Can you work these out from the model? Positions are in its coordinate system, mm. Face numbers are marked on the shaded views. A direction names the side the tool comes from. Give positions to 0.01 mm unless a question says otherwise; leave off trailing zeros. Loops run counter-clockwise (first coordinate to the right, second up) from the corner with the lowest first, then second, coordinate; pieces in that order, holes last. Notation, with made-up numbers: (22.5, -11) - (44.5, -11) arc R14 cw to (44.5, 13) - close; hole circle Ø5 at (42.5, 7.5). An arc over 180 degrees is marked (long way). Answer as a JSON object with one key per item and string values. Group by question number.
Item 1: Suppose I cut it at C-C on z = 147.6. Write out the boundary of the cut face in (x, y), and give its area (3 significant figures).
Item 2: Suppose I cut it at B-B on x = -35. Write out the boundary of the cut face in (y, z), and give its area (3 significant figures).
Item 3: Which directions (+Z, -Z, +X, -X, +Y, -Y) give clear straight access to the entire face, cutting with the end or side of a thin tool? Please do the marked faces 5, 6, 7, 8 and 9.
Item 4: Suppose I cut it at D-D on x = -28. Write out the boundary of the cut face in (y, z).
Item 5: Please list where these lines run through material, in increasing order: L1, parallel to Z at x = -28, y = 12.5; L2, parallel to Z at x = -42, y = 10; L3, parallel to X at y = 10, z = 139.
Item 6: Will these pins go through, and if not, where does the flat tip stop? pin 1 (3 mm diameter, centred on x = -50.5, z = 117.5, fed in from -Y); pin 2 (4 mm diameter, centred on x = -29, y = -11.5, fed in from +Z); pin 3 (1.8 mm diameter, centred on x = -33.5, z = 96, fed in from +Y); pin 4 (2.5 mm diameter, centred on x = -28, z = 163.6, fed in from -Y).
Item 7: Thinking about a two-plate mould opening in X: for the marked faces 1, 2, 3 and 4, which applies, pulls with the +X half, pulls with the -X half, needs draft (parallel to the pull), parting line crosses it, or undercut?
Item 8: Suppose I cut it at A-A on y = -7. Write out the boundary of the cut face in (x, z).
Autodesk Inventor part; units mm, degrees
ref_plane "YZ Plane" through (0, 0, 0) normal (1, 0, 0) x (0, 1, 0)
ref_plane "XZ Plane" through (0, 0, 0) normal (0, 1, 0) x (-1, 0, 0)
ref_plane "XY Plane" through (0, 0, 0) normal (0, 0, 1) x (1, 0, 0)
sketch "Sketch1" plane through (0, 0, 0) normal (0, 1, 0) x (-1, 0, 0)
  line L0 (0, 0) -> (0, 62)
  line L1 (0, 62) -> (70, 62)
  line L2 (70, 62) -> (70, 0)
  line L3 (76, 0) -> (76, 68)
  line L4 (76, 68) -> (-6, 68)
  line L5 (-6, 68) -> (-6, 0)
  line L6 (70, 0) -> (76, 0)
  line L7 (-6, 0) -> (0, 0)
  dimension "d0" = 62
  dimension "d1" = 70
  dimension "d2" = 6
  dimension "d5" = 62
extrude "Extrusion1" add sketch "Sketch1" along normal blind 40
sketch "Sketch2" plane through (6, 0, 68) normal (1, 0, 0) x (0, 0, -1)
  line L0 (68, 0) -> (68, 40)
  circle A0 centre (56, 25) radius 1.5
  circle A1 centre (51, 20) radius 1.5
  circle A2 centre (56, 15) radius 1.5
  circle A3 centre (61, 20) radius 1.5
  point P0 (56, 20)
  dimension "d9" = 3
  dimension "d12" = 360
extrude "Extrusion2" cut sketch "Sketch2" against normal up to surface (6 mm away)
sketch "Sketch3" plane through (-70, 0, 62) normal (1, 0, 0) x (0, 0, -1)
  line L0 (62, 0) -> (62, 40)
  line L1 (62, 20) -> (58, 20)
  circle A0 centre (50, 20) radius 5.75
  dimension "d16" = 4
  dimension "d18" = 11.5
extrude "Extrusion3" add sketch "Sketch3" along normal blind 5
fillet "Fillet1" radius 8 4 edges at (3, 40, 0) (3, 0, 0) (-73, 0, 0) (-73, 40, 0)
sketch "Sketch4" plane through (-76, 0, 68) normal (0, 0, 1) x (1, 0, 0)
  line L0 (41, 0) -> (41, 20)
  line L1 (30, 0) -> (30, 40)
  line L2 (76, 40) -> (6, 40)
  line L3 (52, 0) -> (52, 40)
  line L4 (25, 0) -> (25, 40)
  line L5 (57, 0) -> (57, 40)
  line L6 (25, 40) -> (30, 40)
  line L7 (52, 40) -> (57, 40)
  line L8 (52, 0) -> (57, 0)
  line L9 (76, 0) -> (6, 0)
  line L10 (30, 0) -> (25, 0)
  dimension "d22" = 11
  dimension "d23" = 11
  dimension "d24" = 5
  dimension "d25" = 5
extrude "Extrusion4" add sketch "Sketch4" along normal blind 24 contours L9 L4 L2 L1 | L2 L5 L8 L3
sketch "Sketch5" plane through (-76, 0, 92) normal (0, 0, 1) x (1, 0, 0)
  line L0 (25, 0) -> (25, 40)
  line L1 (57, 0) -> (57, 40)
  line L2 (25, 0) -> (57, 0)
  line L3 (57, 0) -> (57, 40)
  line L4 (52, 0) -> (52, 40)
  line L5 (57, 40) -> (52, 40)
  line L6 (30, 0) -> (52, 0)
  line L7 (41, 3.3) -> (41, 9.3)
  line L8 (41, 9.3) -> (52, 9.3)
  line L9 (41, 9.3) -> (30, 9.3)
  line L10 (52, 9.3) -> (52, 40)
  line L11 (76, 40) -> (6, 40)
  line L12 (30, 40) -> (30, 0)
  line L13 (30, 9.3) -> (30, 40)
  line L14 (30, 40) -> (25, 40)
  line L15 (25, 40) -> (25, 0)
  line L16 (76, 0) -> (6, 0)
  dimension "d29" = 6
extrude "Extrusion5" add sketch "Sketch5" along normal blind 6 contours L0 L11 L12 L2 | L12 L9 L8 L4 L2 | L4 L5 L1 L2
sketch "Sketch6" plane through (-76, 0, 98) normal (0, 0, 1) x (1, 0, 0)
  line L0 (25, 0) -> (25, 40)
  line L1 (25, 40) -> (25, 0)
  line L2 (57, 40) -> (57, 0)
  line L3 (25, 0) -> (57, 0)
  line L4 (57, 0) -> (57, 40)
  line L5 (52, 0) -> (52, 40)
  line L6 (57, 40) -> (52, 40)
  line L7 (30, 40) -> (25, 40)
  line L8 (25, 40) -> (30, 40)
  line L9 (30, 0) -> (52, 0)
  line L10 (30, 40) -> (30, 0)
  line L11 (30, 0) -> (52, 0)
  line L12 (52, 40) -> (52, 9.3)
  line L13 (52, 40) -> (52, 0)
  line L14 (25, 0) -> (57, 0)
  point P0 (76, 0)
extrude "Extrusion6" add sketch "Sketch6" along normal blind 13.8
sketch "Sketch8" plane through (-76, 0, 111.8) normal (0, 0, 1) x (1, 0, 0)
  line L0 (52, 9.3) -> (30, 9.3)
  arc A0 (30.0455, 19.3) -> (51.9545, 19.3) centre (41, 20.3) ccw
  line L1 (51.9545, 19.3) -> (52, 19.3)
  line L2 (52, 0) -> (52, 40)
  line L3 (30, 40) -> (52, 40)
  line L4 (52, 19.3) -> (52, 40)
  line L5 (57, 40) -> (52, 40)
  line L6 (52, 40) -> (57, 40)
  line L7 (57, 40) -> (57, 6.3)
  line L8 (57, 40) -> (57, 0)
  line L9 (57, 6.3) -> (25, 6.3)
  line L10 (25, 0) -> (25, 40)
  line L11 (0, 40) -> (25, 40)
  line L12 (25, 6.3) -> (25, 40)
  line L13 (25, 40) -> (30, 40)
  line L14 (30, 40) -> (30, 19.3)
  line L15 (30, 40) -> (30, 0)
  line L16 (30, 19.3) -> (30.0455, 19.3)
  point P0 (76, 0)
  dimension "d37" = 33.7
  dimension "d38" = 11
extrude "Extrusion7" add sketch "Sketch8" along normal blind 13.8 contours L2 L9 L15 L0 | L0 A0 L1 L2 | L2 L5 L7 L9 | L0 L15 L16 A0 | L15 L9 L10 L13 L14
sketch "Sketch9" plane through (-76, 0, 125.6) normal (0, 0, 1) x (1, 0, 0)
  line L0 (25, 6.3) -> (57, 6.3)
  arc A0 (30.0455, 19.3) -> (51.9545, 19.3) centre (41, 20.3) ccw
  arc A1 (38, 20.3) -> (44, 20.3) centre (41, 20.3) ccw
  line L1 (25, 40) -> (25, 6.3)
  line L2 (25, 6.3) -> (25, 40)
  line L3 (57, 6.3) -> (57, 40)
  line L4 (25, 40) -> (57, 40)
  line L5 (38, 20.3) -> (30, 20.3)
  line L6 (30, 19.3) -> (30, 40)
  line L7 (44, 20.3) -> (52, 20.3)
  line L8 (52, 40) -> (52, 20.3)
  line L9 (52, 40) -> (57, 40)
  line L10 (57, 40) -> (57, 6.3)
  line L11 (57, 6.3) -> (25, 6.3)
  point P0 (76, 0)
  dimension "d41" = 6
extrude "Extrusion8" add sketch "Sketch9" along normal blind 50 contours L1 L4 L6 L5 A1 L7 L8 L3 L0
sketch "Sketch10" plane through (0, 40, 0) normal (0, 1, 0) x (1, 0, 0)
  line L0 (-24, -98) -> (-46, -98)
  line L1 (-46, -98) -> (-24, -98)
  line L2 (-24, -175.6) -> (-46, -175.6)
  line L3 (-19, -68) -> (-19, -175.6)
  line L4 (-19, -175.6) -> (-24, -175.6)
  line L5 (-24, -175.6) -> (-24, -98)
  line L6 (-24, -98) -> (-19, -98)
  line L7 (-19, -98) -> (-19, -175.6)
  line L8 (-51, -175.6) -> (-19, -175.6)
  line L9 (-51, -175.6) -> (-46, -175.6)
  line L10 (-46, -98) -> (-51, -98)
  line L11 (-51, -98) -> (-51, -175.6)
  point P0 (0, 0)
extrude "Extrusion9" cut sketch "Sketch10" against normal up to surface (19.7 mm away)
sketch "Sketch11" plane through (-76, 0, 175.6) normal (0, 0, 1) x (1, 0, 0)
  arc A0 (38, 20.3) -> (44, 20.3) centre (41, 20.3) ccw
  line L0 (52, 20.3) -> (44, 20.3)
  arc A1 (19.7397, 20.3) -> (62.2603, 20.3) centre (41, 20.3) ccw
  arc A2 (38, 20.3) -> (44, 20.3) centre (41, 20.3) ccw
  line L1 (19.7397, 20.3) -> (38, 20.3)
  line L2 (44, 20.3) -> (62.2603, 20.3)
  point P0 (76, 0)
extrude "Extrusion10" add sketch "Sketch11" along normal blind 36
sketch "Sketch12" plane through (-76, 0, 211.6) normal (0, 0, 1) x (1, 0, 0)
  arc A0 (38, 20.3) -> (44, 20.3) centre (41, 20.3) ccw
  circle A1 centre (41, 20.3) radius 19
  point P0 (76, 0)
  dimension "d49" = 38
extrude "Extrusion11" cut sketch "Sketch12" against normal blind 32
sketch "Sketch13" plane through (-76, 0, 211.6) normal (0, 0, 1) x (1, 0, 0)
  line L0 (62.2603, 20.3) -> (57, 20.3)
  arc A0 (19.7397, 20.3) -> (62.2603, 20.3) centre (41, 20.3) ccw
  line L1 (22, 20.3) -> (38, 20.3)
  arc A1 (22, 20.3) -> (60, 20.3) centre (41, 20.3) ccw
  arc A2 (22, 20.3) -> (60, 20.3) centre (41, 20.3) ccw
  line L2 (19.7397, 20.3) -> (22, 20.3)
  line L3 (62.2603, 20.3) -> (60, 20.3)
  point P0 (76, 0)
extrude "Extrusion12" add sketch "Sketch13" along normal blind 6.2
fillet "Fillet3" radius 1 5 edges at (-76, 20, 68) (-35, 40, 68) (-6.5, 40, 68) (-63.5, 40, 68) (6, 20, 68)
sketch "Sketch20" plane through (-19, 0, 111.8) normal (1, 0, 0) x (0, 0, -1)
  line L0 (0, 6.3) -> (-63.8, 6.3)
  line L1 (0, 6.3) -> (0, 0)
  line L2 (-63.8, 6.3) -> (0, 6.3)
  line L3 (0, 6.3) -> (0, 0)
  line L4 (0, 0) -> (-63.8, 0)
  line L5 (-63.8, 0) -> (-63.8, 6.3)
  point P0 (111.8, 0)
extrude "Extrusion19" add sketch "Sketch20" against normal up to surface (5 mm away)
sketch "Sketch21" plane through (-51, 0, 68) normal (-1, 0, 0) x (0, 0, 1)
  line L0 (43.8, 6.3) -> (107.6, 6.3)
  line L1 (0, 0) -> (107.6, 0)
  line L2 (43.8, 6.3) -> (107.6, 6.3)
  line L3 (107.6, 6.3) -> (107.6, 0)
  line L4 (107.6, 0) -> (43.8, 0)
  line L5 (43.8, 0) -> (43.8, 6.3)
  point P0 (-68, 0)
  point P1 (107.6, 6.3)
  point P2 (43.8, 0)
extrude "Extrusion20" add sketch "Sketch21" against normal up to surface (5 mm away)
sketch "Sketch22" plane through (-51, 20.3, 98) normal (-1, 0, 0) x (0, 0, 1)
  line L0 (-31, 19.7) -> (0, 19.7)
  line L1 (-31, 19.7) -> (0, 19.7)
  line L2 (0, 0) -> (27.6, 0)
  line L3 (0, 19.7) -> (0, 0)
  line L4 (77.6, 0) -> (119.8, 0)
  line L5 (0, 0) -> (77.6, 0)
  line L6 (-30, -20.3) -> (77.6, -20.3)
  line L7 (77.6, 0) -> (77.6, -20.3)
  line L8 (-31, 19.7) -> (-31, -20.3)
  line L9 (77.6, -20.3) -> (-31, -20.3)
  line L10 (-31, -20.3) -> (-31, 19.7)
  point P0 (-98, -20.3)
extrude "Extrusion21" add sketch "Sketch22" along normal up to surface (5.2603 mm away)
sketch "Sketch23" plane through (-19, 20.3, 98) normal (1, 0, 0) x (0, 0, -1)
  line L0 (31, 19.7) -> (0, 19.7)
  line L1 (0, 19.7) -> (0, 0)
  line L2 (0, 19.7) -> (0, 0)
  line L3 (0, 0) -> (-77.6, 0)
  line L4 (0, 0) -> (-77.6, 0)
  line L5 (-77.6, -20.3) -> (-77.6, -18.1934)
  line L6 (-77.6, 0) -> (-77.6, -20.3)
  line L7 (31, 19.7) -> (31, -20.3)
  line L8 (-77.6, -20.3) -> (31, -20.3)
  line L9 (31, -20.3) -> (31, 19.7)
  line L10 (31, 19.7) -> (0, 19.7)
  point P0 (98, -20.3)
extrude "Extrusion22" add sketch "Sketch23" along normal up to surface (5.2603 mm away)
sketch "Sketch24" plane through (-24, 0, 175.6) normal (0, 0, 1) x (1, 0, 0)
  line L0 (0, 2.1066) -> (0, 0)
  line L1 (0, 20.3) -> (10.2603, 20.3)
  arc A0 (0, 2.1066) -> (10.2603, 20.3) centre (-11, 20.3) ccw
  line L2 (-32.2603, 20.3) -> (-32.2603, 0)
  line L3 (-22, 0) -> (-22, 2.1066)
  arc A1 (-32.2603, 20.3) -> (-22, 2.1066) centre (-11, 20.3) ccw
  line L4 (-32.2603, 20.3) -> (-32.2603, 0)
  line L5 (24, 0) -> (-46, 0)
  line L6 (-22, 0) -> (-32.2603, 0)
  line L7 (-22, 0) -> (-22, 2.1066)
  line L8 (0, 0) -> (0, 2.1066)
  line L9 (10.2603, 39) -> (10.2603, 0)
  line L10 (10.2603, 0) -> (0, 0)
  arc A2 (0, 2.1066) -> (10.2603, 20.3) centre (-11, 20.3) ccw
  line L11 (10.2603, 0) -> (10.2603, 20.3)
extrude "Extrusion23" cut sketch "Sketch24" against normal up to surface (77.6 mm away)
sketch "Sketch25" plane through (-56.2603, 0, 68) normal (-1, 0, 0) x (0, 0, 1)
  line L0 (24, 9.3) -> (24, 0)
  line L1 (24, 0) -> (24, 40)
  line L2 (-1, 40) -> (30, 40)
  line L3 (24, 40) -> (-68, 40)
  line L4 (-68, 8) -> (-68, 32)
  line L5 (-68, 40) -> (-68, 0)
  line L6 (-68, 0) -> (24, 0)
extrude "Extrusion24" cut sketch "Sketch25" along normal mid plane 150
sketch "Sketch26" plane through (-56.2603, 0, 92) normal (-1, 0, 0) x (0, 0, 1)
  line L0 (6, 40) -> (0, 40)
  line L1 (6, 20.3) -> (6, 40)
  line L2 (0, 40) -> (6, 40)
  line L3 (6, 40) -> (6, 20.3)
  line L4 (6, 20.3) -> (0, 20.3)
  line L5 (0, 20.3) -> (0, 40)
  point P0 (-92, 0)
extrude "Extrusion25" cut sketch "Sketch26" against normal up to surface (42.5206 mm away)
sketch "Sketch28" plane through (-46, 6.3, 111.8) normal (0, -1, 0) x (1, 0, 0)
  line L0 (22, 63.8) -> (0, 63.8)
  line L1 (0, 63.8) -> (8, 63.8)
  line L2 (8, 13.8) -> (8, 67.8)
  line L3 (0.0455, 0) -> (21.9545, 0)
  circle A0 centre (18, 28) radius 1.5
  circle A1 centre (18, 35.8) radius 1.5
  circle A2 centre (18, 51.8) radius 1.5
  circle A3 centre (4, 28) radius 1.5
  circle A4 centre (4, 35.8) radius 1.5
  circle A5 centre (4, 51.8) radius 1.5
  point P0 (46, -111.8)
extrude "Extrusion27" cut sketch "Sketch28" against normal through all
sketch "Sketch29" plane through (0, 0, 0) normal (0, -1, 0) x (1, 0, 0)
  line L0 (-24, 98) -> (-46, 98)
  line L1 (-24, 125.6) -> (-24, 92)
  line L2 (-46, 98) -> (-24, 98)
  line L3 (-24, 98) -> (-24, 92)
  line L4 (-24, 92) -> (-46, 92)
  line L5 (-46, 92) -> (-46, 98)
  point P0 (0, 0)
extrude "Extrusion28" cut sketch "Sketch29" against normal up to surface (9.3 mm away)
sketch "Sketch30" plane through (0, 0, 0) normal (0, -1, 0) x (1, 0, 0)
  line L0 (-13.7397, 98) -> (-13.7397, 217.8)
  line L1 (-24, 92) -> (-13.7397, 92)
  line L2 (-13.7397, 98) -> (-24, 98)
  line L3 (-24, 98) -> (-24, 92)
  line L4 (-24, 92) -> (-13.7397, 92)
  line L5 (-13.7397, 92) -> (-13.7397, 98)
  line L6 (-46, 175.6) -> (-46, 98)
  line L7 (-56.2603, 92) -> (-46, 92)
  line L8 (-46, 98) -> (-56.2603, 98)
  line L9 (-56.2603, 98) -> (-56.2603, 92)
  line L10 (-56.2603, 92) -> (-46, 92)
  line L11 (-46, 92) -> (-46, 98)
  point P0 (0, 0)
extrude "Extrusion29" add sketch "Sketch30" along normal blind 18.6
sketch "Sketch31" plane through (0, -18.6, 0) normal (0, -1, 0) x (1, 0, 0)
  line L0 (-13.7397, 98) -> (-24, 98)
  line L1 (-56.2603, 92) -> (-46, 92)
  line L2 (-24, 98) -> (-46, 98)
  line L3 (-46, 98) -> (-46, 92)
  line L4 (-46, 92) -> (-24, 92)
  line L5 (-24, 92) -> (-24, 98)
  point P0 (0, 0)
extrude "Extrusion30" add sketch "Sketch31" against normal blind 9
sketch "Sketch32" plane through (-76, 0, 125.6) normal (0, 0, -1) x (-1, 0, 0)
  line L0 (-44, 20.3) -> (-60, 20.3)
  line L1 (-52, 20.3) -> (-44, 20.3)
  arc A0 (-44, 20.3) -> (-38, 20.3) centre (-41, 20.3) ccw
  line L2 (-38, 20.3) -> (-30, 20.3)
  line L3 (-22, 20.3) -> (-38, 20.3)
  arc A1 (-52, 20.3) -> (-30, 20.3) centre (-41, 20.3) ccw
  arc A2 (-44, 20.3) -> (-38, 20.3) centre (-41, 20.3) ccw
  point P0 (-76, 0)
extrude "Extrusion31" cut sketch "Sketch32" against normal blind 4
properties part number "Tilt_Bracket_Output_2_Lid"
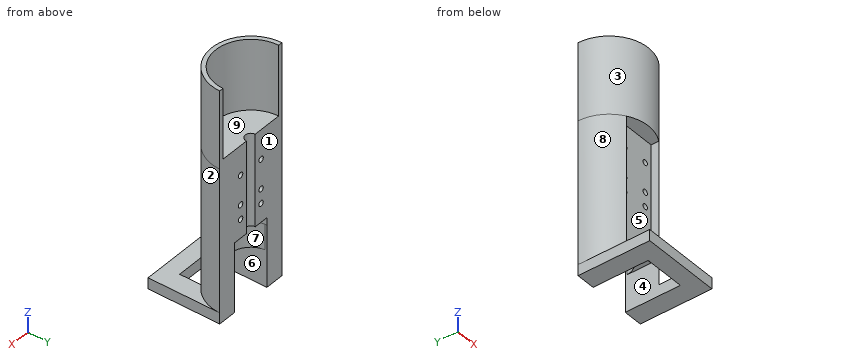
Worked out:
{
 "1": {"outline": "(-56.26, 20.3) arc R21.26 ccw to (-46, 2.11) - (-46, 6.3) - (-43.5, 6.3) - (-43.5, 20.3) - close; (-40.5, 6.3) - (-29.5, 6.3) - (-29.5, 20.3) - (-32, 20.3) arc R3 cw to (-38, 20.3) - (-40.5, 20.3) - close; (-26.5, 6.3) - (-24, 6.3) - (-24, 2.11) arc R21.26 ccw to (-13.74, 20.3) - (-26.5, 20.3) - close", "area": "474 mm2"},
 "2": {"outline": "(-18.6, 92) - (-9.6, 92) - (-9.6, 98) - (-18.6, 98) - close; (-0.96, 175.6) - (6.3, 175.6) - (6.3, 111.8) - (9.3, 111.8) - (9.3, 129.6) - (17.3, 129.6) - (17.3, 179.6) - (1.3, 179.6) - (1.3, 217.8) - (-0.96, 217.8) - close", "area": "773 mm2"},
 "3": {"face 5": "-Z, -Y", "face 6": "-Z", "face 7": "-Z, +Y", "face 8": "+Z, -X, -Y", "face 9": "+Z, +Y"},
 "4": {"outline": "(-18.6, 92) - (-9.6, 92) - (-9.6, 98) - (-18.6, 98) - close; (0.23, 175.6) - (6.3, 175.6) - (6.3, 165.1) - (20.3, 165.1) - (20.3, 179.6) - (2.64, 179.6) - (2.64, 217.8) - (0.23, 217.8) - close; (6.3, 111.8) - (11.81, 111.8) - (11.81, 129.6) - (20.3, 129.6) - (20.3, 138.3) - (6.3, 138.3) - close; (6.3, 141.3) - (20.3, 141.3) - (20.3, 146.1) - (6.3, 146.1) - close; (6.3, 149.1) - (20.3, 149.1) - (20.3, 162.1) - (6.3, 162.1) - close"},
 "5": {"L1": "z = 129.6 to 138.3, 141.3 to 146.1, 149.1 to 162.1, 165.1 to 179.6", "L2": "z = 111.8 to 138.3, 141.3 to 146.1, 149.1 to 162.1, 165.1 to 179.6", "L3": "x = -53.6 to -43.27, -40.73 to -29.27, -26.73 to -16.4"},
 "6": {"pin 1": "stops at y = 4.3", "pin 2": "stops at z = 98", "pin 3": "stops at y = -9.6", "pin 4": "passes through"},
 "7": {"face 1": "needs draft", "face 2": "pulls with the +X half", "face 3": "parting line crosses it", "face 4": "undercut"},
 "8": {"outline": "(-56.26, 92) - (-46, 92) - (-46, 98) - (-56.26, 98) - close; (-24, 92) - (-13.74, 92) - (-13.74, 98) - (-24, 98) - close"}
}
